Model file for the job. Use its own axes, mm. Coordinates: 2 decimals unless noted, no trailing zeros. Write each loop counter-clockwise with the first axis right and the second up, starting at its lowest first coordinate (ties: lowest second). Pieces come first, ordered by that corner, then holes. Notation, with made-up numbers: M 67.25,-30.75 L 80.25,-30.75 A17 ccw 80.25,-26.75 Z; hole C 54,-33 d11. An arc over 180 degrees is marked long. Put each result on its own line as item: value. Start each with the question number.
Q1. Drill centre lines: line 1 along X through (y, z) = (0.95, -6.75); line 2 along Z through (x, y) = (28.5, 2.25); line 3 along X through (y, z) = (1.5, -3.5). Where is each one in solid material? Low to high.
Q2. Cut at B-B (z = -3.5). Write the cut outline in (x, y).
Q3. Cut at D-D (z = 6.5). Write the cut outline in (x, y), then the cut area to 3 significant figures.
Q4. Cut at C-C (y = 0.6). Give the number of separate pieces and of enclosed holes in the cut face, then the cut area to 3 significant figures.
Q5. Cut at A-A (x = 28.5). Write the cut outline in (y, z).
```python
from build123d import *

# Parameters (mm, degrees)
SKETCH_1_W          = 63
SKETCH_1_H          = 21
SKETCH_1_R          = 1.5
EXTRUDE_1_DEPTH     = 3
FILLET_1_R          = 2
SKETCH_3_R          = 1.5
CUT_EXTRUDE_2_DEPTH = 34.339166156


with BuildPart() as part:
    # 草图1 → 凸台-拉伸1 (new body)
    with BuildSketch(Plane(origin=(0, 0, 0), x_dir=(1, 0, 0), z_dir=(0, 1, 0))):
        Rectangle(SKETCH_1_W, SKETCH_1_H)
        with Locations(Location((-11.69, 6.75, 0), (0, 0, 270))):
            Circle(SKETCH_1_R, mode=Mode.SUBTRACT)
        with Locations(Location((11.69, 6.75, 0), (0, 0, 270))):
            Circle(SKETCH_1_R, mode=Mode.SUBTRACT)
        with Locations(Location((11.69, -6.75, 0), (0, 0, 270))):
            Circle(SKETCH_1_R, mode=Mode.SUBTRACT)
        with Locations(Location((-11.69, -6.75, 0), (0, 0, 270))):
            Circle(SKETCH_1_R, mode=Mode.SUBTRACT)
    extrude(amount=EXTRUDE_1_DEPTH)

    # 圆角1
    fillet_1_edges = [part.edges().sort_by_distance(p)[0] for p in [
        (31.5, 1.5, 10.5),
        (-31.5, 1.5, 10.5),
        (-31.5, 1.5, -10.5),
        (31.5, 1.5, -10.5),
    ]]
    fillet(fillet_1_edges, radius=FILLET_1_R)

    # 草图3 → 切除-拉伸2 (cut, through all)
    with BuildSketch(Plane(origin=(0, 3, 0), x_dir=(1, 0, 0), z_dir=(0, 1, 0))):
        with Locations(Location((-28.5, -6.5, 0), (0, 0, 270))):
            Circle(SKETCH_3_R)
        with Locations(Location((-28.5, 3.5, 0), (0, 0, 270))):
            Circle(SKETCH_3_R)
        with Locations(Location((28.5, -6.5, 0), (0, 0, 90))):
            Circle(SKETCH_3_R)
        with Locations(Location((28.5, 3.5, 0), (0, 0, 90))):
            Circle(SKETCH_3_R)
    extrude(amount=-CUT_EXTRUDE_2_DEPTH, mode=Mode.SUBTRACT)


solid = part.part
```
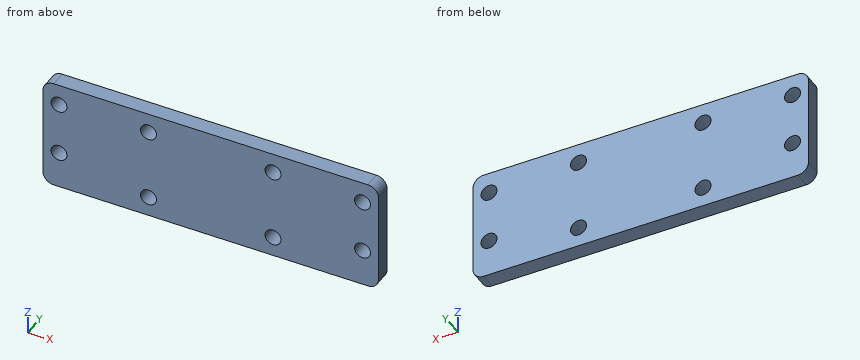
Computed values:
1. line 1: -31.5 to -13.19, -10.19 to 10.19, 13.19 to 31.5
1. line 2: -10.5 to -5, -2 to 5, 8 to 10.5
1. line 3: -31.5 to -30, -27 to 27, 30 to 31.5
2. outline: M -31.5,0 L -30,0 L -30,3 L -31.5,3 Z; M -27,0 L 27,0 L 27,3 L -27,3 Z; M 30,0 L 31.5,0 L 31.5,3 L 30,3 Z
3. outline: M -31.5,0 L -30,0 L -30,3 L -31.5,3 Z; M -27,0 L -13.17,0 L -13.17,3 L -27,3 Z; M -10.21,0 L 10.21,0 L 10.21,3 L -10.21,3 Z; M 13.17,0 L 27,0 L 27,3 L 13.17,3 Z; M 30,0 L 31.5,0 L 31.5,3 L 30,3 Z
3. area: 153 mm2
4. separate pieces: 1
4. enclosed holes: 8
4. area: 1,260 mm2
5. outline: M 0,-10.5 L 3,-10.5 L 3,-5 L 0,-5 Z; M 0,-2 L 3,-2 L 3,5 L 0,5 Z; M 0,8 L 3,8 L 3,10.5 L 0,10.5 Z
